from build123d import *

# Parameters (mm, degrees)
SKETCH1_W           = 12.573
SKETCH1_H           = 6.35
BOSS_EXTRUDE1_DEPTH = 6.35


with BuildPart() as part:
    # Sketch1 → Boss-Extrude1 (new body)
    with BuildSketch(Plane.XY):
        Polygon((0, 0), (12.573, 0), (12.573, 6.35), (25.527, 6.35), (25.527, 0), (266.573, 0), (266.573, 6.35), (279.527, 6.35), (279.527, 0), (292.1, 0), (292.1, -12.827), (285.75, -12.827), (285.75, -25.273), (292.1, -25.273), (292.1, -38.227), (285.75, -38.227), (285.75, -50.673), (292.1, -50.673), (292.1, -63.627), (285.75, -63.627), (285.75, -76.073), (292.1, -76.073), (292.1, -89.027), (285.75, -89.027), (285.75, -101.473), (292.1, -101.473), (292.1, -114.427), (285.75, -114.427), (285.75, -126.873), (292.1, -126.873), (292.1, -139.827), (285.75, -139.827), (285.75, -152.273), (292.1, -152.273), (292.1, -165.227), (285.75, -165.227), (285.75, -177.673), (292.1, -177.673), (292.1, -190.627), (285.75, -190.627), (285.75, -203.073), (292.1, -203.073), (292.1, -216.027), (285.75, -216.027), (285.75, -228.473), (292.1, -228.473), (292.1, -241.427), (285.75, -241.427), (285.75, -253.873), (292.1, -253.873), (292.1, -266.827), (285.75, -266.827), (285.75, -279.273), (292.1, -279.273), (292.1, -292.227), (285.75, -292.227), (285.75, -304.673), (292.1, -304.673), (292.1, -317.627), (285.75, -317.627), (285.75, -330.073), (292.1, -330.073), (292.1, -342.9), (279.273, -342.9), (279.273, -336.55), (266.827, -336.55), (266.827, -342.9), (253.873, -342.9), (253.873, -336.55), (241.427, -336.55), (241.427, -342.9), (228.473, -342.9), (228.473, -336.55), (216.027, -336.55), (216.027, -342.9), (203.073, -342.9), (203.073, -336.55), (190.627, -336.55), (190.627, -342.9), (177.673, -342.9), (177.673, -336.55), (165.227, -336.55), (165.227, -342.9), (152.273, -342.9), (152.273, -336.55), (139.827, -336.55), (139.827, -342.9), (126.873, -342.9), (126.873, -336.55), (114.427, -336.55), (114.427, -342.9), (101.473, -342.9), (101.473, -336.55), (89.027, -336.55), (89.027, -342.9), (76.073, -342.9), (76.073, -336.55), (63.627, -336.55), (63.627, -342.9), (50.673, -342.9), (50.673, -336.55), (38.227, -336.55), (38.227, -342.9), (25.273, -342.9), (25.273, -336.55), (12.827, -336.55), (12.827, -342.9), (0, -342.9), (0, -330.073), (6.35, -330.073), (6.35, -317.627), (0, -317.627), (0, -304.673), (6.35, -304.673), (6.35, -292.227), (0, -292.227), (0, -279.273), (6.35, -279.273), (6.35, -266.827), (0, -266.827), (0, -253.873), (6.35, -253.873), (6.35, -241.427), (0, -241.427), (0, -228.473), (6.35, -228.473), (6.35, -216.027), (0, -216.027), (0, -203.073), (6.35, -203.073), (6.35, -190.627), (0, -190.627), (0, -177.673), (6.35, -177.673), (6.35, -165.227), (0, -165.227), (0, -152.273), (6.35, -152.273), (6.35, -139.827), (0, -139.827), (0, -126.873), (6.35, -126.873), (6.35, -114.427), (0, -114.427), (0, -101.473), (6.35, -101.473), (6.35, -89.027), (0, -89.027), (0, -76.073), (6.35, -76.073), (6.35, -63.627), (0, -63.627), (0, -50.673), (6.35, -50.673), (6.35, -38.227), (0, -38.227), (0, -25.273), (6.35, -25.273), (6.35, -12.827), (0, -12.827), align=None)
        Polygon((260.870458318, -155.351665797), (248.363399855, -157.556997654), (247.842941537, -154.605331856), (260.35, -152.4), align=None, mode=Mode.SUBTRACT)
        Polygon((235.856341392, -159.76232951), (223.349282928, -161.967661366), (222.82882461, -159.015995569), (235.335883073, -156.810663713), align=None, mode=Mode.SUBTRACT)
        with Locations((158.75, -130.81)):
            Rectangle(SKETCH1_W, SKETCH1_H, mode=Mode.SUBTRACT)
        with Locations((133.35, -130.81)):
            Rectangle(SKETCH1_W, SKETCH1_H, mode=Mode.SUBTRACT)
        Polygon((210.842224465, -164.172993223), (198.335166002, -166.378325079), (197.814707684, -163.426659282), (210.321766147, -161.221327425), align=None, mode=Mode.SUBTRACT)
        Polygon((185.828107539, -168.583656936), (173.321049075, -170.788988792), (172.800590757, -167.837322995), (185.30764922, -165.631991138), align=None, mode=Mode.SUBTRACT)
        Polygon((160.813990612, -172.994320648), (148.306932149, -175.199652505), (147.786473831, -172.247986707), (160.293532294, -170.042654851), align=None, mode=Mode.SUBTRACT)
        Polygon((135.799873686, -177.404984361), (123.292815222, -179.610316217), (122.772356904, -176.65865042), (135.279415367, -174.453318564), align=None, mode=Mode.SUBTRACT)
        Polygon((110.785756759, -181.815648074), (98.278698296, -184.02097993), (97.758239978, -181.069314133), (110.265298441, -178.863982276), align=None, mode=Mode.SUBTRACT)
    extrude(amount=BOSS_EXTRUDE1_DEPTH)


solid = part.part
Check sheet for the modelled part. Datum: model origin and axes. Units: mm. Give positions to 0.01 mm unless a question says otherwise; leave off trailing zeros. Write each loop counter-clockwise with the first axis right and the second up, starting at its lowest first coordinate (ties: lowest second). Pieces come first, ordered by that corner, then holes. Notation, with made-up numbers: (-23, 58) -> (-1, 58) arc R26 ccw to (-1, 78) -> close; hole circle Ø6 at (-7.75, -31.5). An arc over 180 degrees is marked (long way). Use one line per item in the form item = value. Start each with the question number.
1. Section check B-B (z = 5). Count the separate pieces of the cut face and the enclosed holes in it, and give its area (3 significant figures).
2. Go/stop test with flat-tipped pins: P1, Ø1.9, axis at x = 249.5, z = 2.5, coming from the -Y side; P2, Ø3, axis at x = 290, z = 4, coming from the +Y side; P3, Ø1.9, axis at y = -144, z = 4.5, coming from the -X side. Record where each tip stops, or that it passes through.
3. Section check A-A (y = -246.5). Record the cut outline in (x, z), and give its area (3 significant figures).
4. Thickness scan on line 1 along X through (y, z) = (-131.5, 3); line 2 along Y through (x, z) = (155.5, 3) (3 decimals); line 3 along Y through (x, z) = (132.5, 4.25) (3 decimals). Record the ranges inside material, lowest first. Write a range as from..to.
Conclusion:
q1.separate_pieces = 1
q1.enclosed_holes = 9
q1.area = 97,000 mm²
q2.P1 = -336.55
q2.P2 = 0
q2.P3 = 6.35
q3.outline = (6.35, 0) -> (285.75, 0) -> (285.75, 6.35) -> (6.35, 6.35) -> close
q3.area = 1,770 mm²
q4.line_1 = 0..127.06, 139.64..152.46, 165.04..292.1
q4.line_2 = -342.9..-173.931, -170.888..-133.985, -127.635..0
q4.line_3 = -342.9..-177.987, -174.943..-133.985, -127.635..0
